Could you check a few things on this model? Use its own coordinates, in mm. A direction names the side the tool comes from. Round coordinates to 2 decimals unless told otherwise and drop trailing zeros. Loops run counter-clockwise (first coordinate to the right, second up) from the corner with the lowest first, then second, coordinate; pieces in that order, holes last. Notation, with made-up numbers: M -39.5,72.5 L 12.5,72.5 A28 cw 12.5,94.5 Z; hole C -16.5,-17.75 d9. An arc over 180 degrees is marked long. Return JSON: item names as keys, results as strings. Group by question number.
```python
from build123d import *

# Parameters (mm, degrees)
F1_DEPTH = 21.43125
F2_R     = 9.525
F3_DEPTH = 50.8
F4_R     = 1.5875
F5_DEPTH = 42.8635


with BuildPart() as f1:
    # F0 (on Right) → F1 (new body, symmetric)
    with BuildSketch(Plane.YZ):
        Polygon((-152.4, 69.85), (-152.4, 0), (152.4, 0), (152.4, 19.05), align=None)
    extrude(amount=F1_DEPTH, both=True)

    # F2 (on face) → F3 (cut)
    with BuildSketch(Plane.XZ.offset(152.4)):
        with Locations((0, 34.925)):
            Circle(F2_R)
    extrude(amount=-F3_DEPTH, mode=Mode.SUBTRACT)

    # F4 (on face) → F5 (intersect, through all)
    with BuildSketch(Plane.YZ.offset(21.43125)):
        Polygon((-73.0092376471, 55.0932995975), (-152.4, 55.0932995975), (-152.4, 0), (112.9424795508, 0), (63.7318268418, 24.0341164172), (-73.0092376471, 24.0341164172), (-73.0092376471, 37.3451933265), align=None)
        with Locations((-139.1612589359, 9.525)):
            Circle(F4_R, mode=Mode.SUBTRACT)
        with Locations((51.7203733325, 9.525)):
            Circle(F4_R, mode=Mode.SUBTRACT)
    extrude(amount=-F5_DEPTH, mode=Mode.INTERSECT)


solid = f1.part
```
1. If we section it at A-A, the plane x = -16: Please give me the cut outline in (y, z) (1 decimal).
2. If we section it at C-C, the plane y = -52: Please give me the cut outline in (x, z), then the cut area to 3 significant figures.
3. We'd pull the mould along X, two halves only. Please class faces 1 (the face through (-1.24, -127.36, 44.37)), 2 (the face through (0, -73.009, 39)), 3 (the face through (21.431, -51, 22)): +X half, -X half, draft (parallel to the pull), parting line (faces both ways), or undercut.
4. On a 3-axis mill with a long thin cutter (end or side, diameter ignored), from which of +Z, -Z, +X, -X, +Y, -Y can I reach the whole of each face in a straight line? I mean faces 4 (the face through (0, -152.4, 22)), 5 (the face through (0, -4, 24.034)), 6 (the face through (0, -101.6, 35)). Say none if no direction works.
5. I'm going to push flat-ended pins straight in: pin 1 Ø9.5 at (x, z) = (-3.5, 44) entering from +Y; pin 2 Ø4 at (x, y) = (-0.5, -75.5) entering from -Z; pin 3 Ø3 at (x, z) = (-13, 14) entering from +Y; pin 4 Ø1.9 at (y, z) = (51.72, 9.52) entering from -X. Where does each tip first touch, or does it pass through?
6. If we section it at D-D, the plane z = 39.5: Please give me the cut outline in (x, y), then the cut area to 3 significant figures.
7. I need wall thicknesses on probe 1 along Z at (x, y) = (0, -137); probe 2 along Y at (x, z) = (17.5, 28); probe 3 along Z at (x, y) = (-19, -8). Which ranges of each line are inside material? Lowest first, please.
8. If we section it at B-B, the plane x = 0: Give the number of separate pieces and of enclosed holes in the cut face, then the cut area to 3 significant figures.
Geometry results:
{
 "1": {"outline": "M -152.4,0 L 112.9,0 L 63.7,24 L -73,24 L -73,55.1 L -152.4,55.1 Z; hole C -139.2,9.5 d3.2; hole C 51.7,9.5 d3.2"},
 "2": {"outline": "M -21.43,0 L 21.43,0 L 21.43,24.03 L -21.43,24.03 Z", "area": "1,030 mm^2"},
 "3": {"face 1": "undercut", "face 2": "draft", "face 3": "+X half"},
 "4": {"face 4": "+Z, -Z, +X, -X, -Y", "face 5": "+Z, +X, -X, +Y", "face 6": "-Y"},
 "5": {"pin 1": "y = -73.01", "pin 2": "z = 0", "pin 3": "y = 87.35", "pin 4": "through"},
 "6": {"outline": "M -21.43,-152.4 L -8.35,-152.4 L -8.35,-101.6 L 8.35,-101.6 L 8.35,-152.4 L 21.43,-152.4 L 21.43,-73.01 L -21.43,-73.01 Z", "area": "2,550 mm^2"},
 "7": {"probe 1": "0 to 25.4, 44.45 to 55.09", "probe 2": "-152.4 to -73.01", "probe 3": "0 to 24.03"},
 "8": {"separate pieces": "1", "enclosed holes": "2", "area": "7,270 mm^2"}
}
